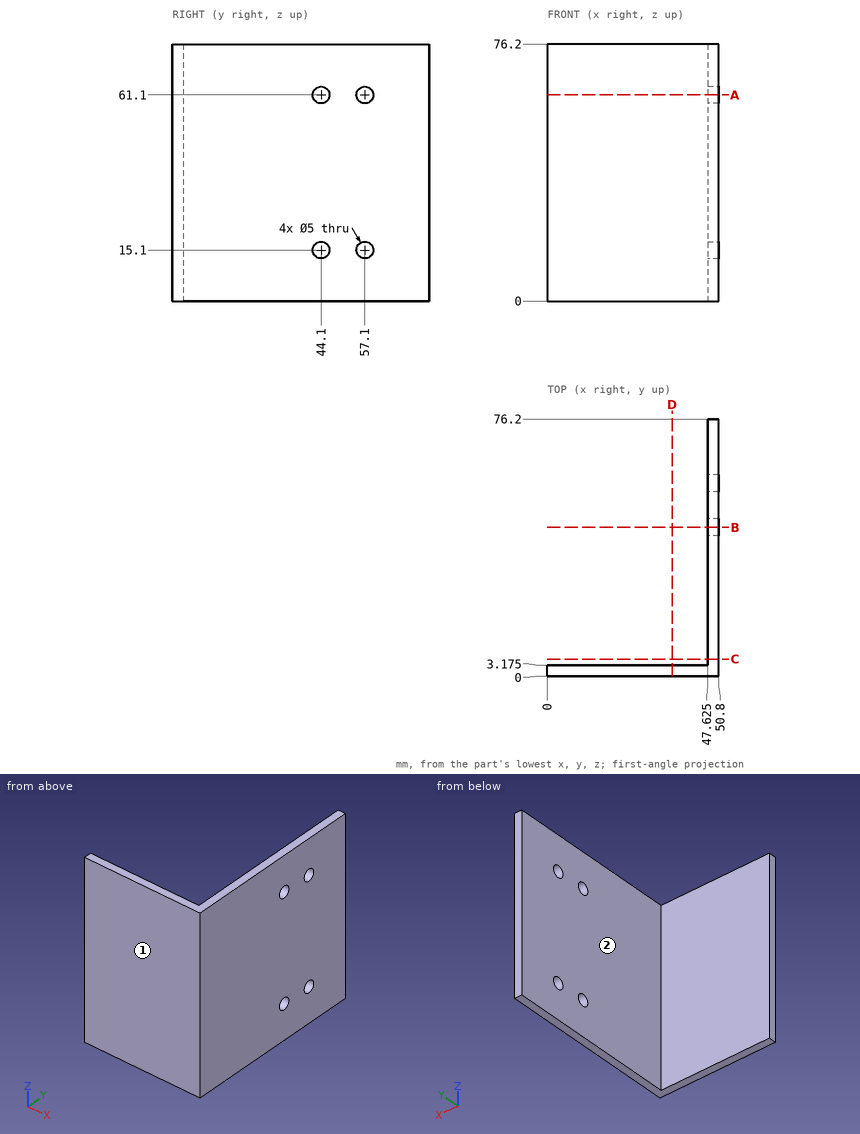
Answer from the drawing. Dimensions are ordinates in mm from the lowest x, y and z of the part. A direction names the side the tool comes from. Coordinates: 2 decimals unless noted, no trailing zeros. Write each loop counter-clockwise with the first axis right and the second up, starting at its lowest first coordinate (ties: lowest second). Pieces come first, ordered by that corner, then holes. Notation, with made-up numbers: M 75.5,27 L 125.5,27 A25 cw 125.5,49 Z; hole C 35,-21.5 d5. An arc over 180 degrees is marked long. Use a Markdown table: item, result.
Q1. The part is cut by section A-A, the plane z = 61.1. Write down the section's boundary in (x, y) (3 decimals), then the cut area to 3 significant figures.
Answer block:
| item | result |
|---|---|
| outline | M 0,0 L 50.8,0 L 50.8,41.6 L 47.625,41.6 L 47.625,3.175 L 0,3.175 Z; M 47.625,46.6 L 50.8,46.6 L 50.8,54.6 L 47.625,54.6 Z; M 47.625,59.6 L 50.8,59.6 L 50.8,76.2 L 47.625,76.2 Z |
| area | 361 mm2 |
Q2. Straight lines are drawn through the part: L1, parallel to Y at x = 49.4, z = 15.1; L2, parallel to Z at x = 48, y = 57; L3, parallel to X at y = 30, z = 55 (3 decimals). For each, find the intervals that lie inside material, in ascending order. Write a range as [from, to].
Answer block:
| item | result |
|---|---|
| L1 | y = [0, 41.6], [46.6, 54.6], [59.6, 76.2] |
| L2 | z = [0, 12.6], [17.6, 58.6], [63.6, 76.2] |
| L3 | x = [47.625, 50.8] |
Q3. The part is cut by section B-B, the plane y = 44.1. Write down the section's boundary in (x, z) (3 decimals).
Answer block:
| item | result |
|---|---|
| outline | M 47.625,0 L 50.8,0 L 50.8,12.6 L 47.625,12.6 Z; M 47.625,17.6 L 50.8,17.6 L 50.8,58.6 L 47.625,58.6 Z; M 47.625,63.6 L 50.8,63.6 L 50.8,76.2 L 47.625,76.2 Z |
Q4. Which of the six approach directions +Z, -Z, +X, -X, +Y, -Y give full straight-line access (tool end or side, diameter ignored) to the marked faces 1 and 2?
Answer block:
| item | result |
|---|---|
| face 1 | +Z, -Z, +X, -X, -Y |
| face 2 | +Z, -Z, -X, +Y |
Q5. Each of these flat-tipped pins is pushed along its axis until it touches: pin 1 Ø12 at (x, z) = (38, 41.5) entering from +Y (3 decimals); pin 2 Ø22 at (y, z) = (41, 24.5) entering from -X (3 decimals). Where does it stop, or does it pass through?
Answer block:
| item | result |
|---|---|
| pin 1 | stops at y = 3.175 |
| pin 2 | stops at x = 47.625 |
Q6. The part is cut by section C-C, the plane y = 5. Write down the section's boundary in (x, z) (3 decimals), then the cut area to 3 significant figures.
Answer block:
| item | result |
|---|---|
| outline | M 47.625,0 L 50.8,0 L 50.8,76.2 L 47.625,76.2 Z |
| area | 242 mm2 |
Q7. The part is cut by section D-D, the plane x = 37. Write down the section's boundary in (y, z) (3 decimals).
Answer block:
| item | result |
|---|---|
| outline | M 0,0 L 3.175,0 L 3.175,76.2 L 0,76.2 Z |
